Source: CAD feature listing. Evaluate the final solid. Frame: model axes, mm. A direction names the side the tool comes from. Give positions to 0.01 mm unless a question says otherwise; leave off trailing zeros. Write each loop counter-clockwise with the first axis right and the second up, starting at its lowest first coordinate (ties: lowest second). Pieces come first, ordered by that corner, then holes. Notation, with made-up numbers: (9.5, -24) -> (65.5, -24) arc R29 ccw to (65.5, 4) -> close; hole circle Ø7 at (-23, -13). An arc over 180 degrees is marked (long way). Write item = value, one per line.
from build123d import *

# Parameters (mm, degrees)
BOSS_EXTRUDE1_DEPTH = 10
SKETCH2_R           = 5
BOSS_EXTRUDE2_DEPTH = 30
CUT_EXTRUDE1_START  = 3.5
CUT_EXTRUDE1_DEPTH  = 4.5
CHAMFER1_SIZE       = 0.5


with BuildPart() as part:
    # Sketch1 → Boss-Extrude1 (new body)
    with BuildSketch(Plane.XY):
        with BuildLine():
            Line((-2, 7), (2, 7))
            Line((2, 7), (2, 4.582575695))
            ThreePointArc((2, 4.582575695), (0, -5), (-2, 4.582575695))
            Line((-2, 4.582575695), (-2, 7))
        make_face()
    extrude(amount=BOSS_EXTRUDE1_DEPTH)

    # Sketch2 → Boss-Extrude2 (add)
    with BuildSketch(Plane.XY.offset(10)):
        Circle(SKETCH2_R)
    extrude(amount=BOSS_EXTRUDE2_DEPTH)

    # Sketch3 → Cut-Extrude1 (cut, through all)
    with BuildSketch(Plane(origin=(0, 0, 0), x_dir=(1, 0, 0), z_dir=(0, 1, 0)).offset(CUT_EXTRUDE1_START)):
        with BuildLine():
            Line((1.5, -30), (1.5, -35))
            ThreePointArc((1.5, -35), (0, -36.5), (-1.5, -35))
            Line((-1.5, -35), (-1.5, -30))
            ThreePointArc((-1.5, -30), (0, -28.5), (1.5, -30))
        make_face()
    extrude(amount=CUT_EXTRUDE1_DEPTH, mode=Mode.SUBTRACT)

    # Chamfer1
    chamfer1_edges = [part.edges().sort_by_distance(p)[0] for p in [
        (-5, 0, 40),
    ]]
    chamfer(chamfer1_edges, length=CHAMFER1_SIZE)


solid = part.part
(1) Section query D-D (z = 32). Return loops of the section in (x, y).
Values follow:
outline = (-1.5, 3.5) -> (-1.5, 4.77) arc R5 ccw (long way) to (1.5, 4.77) -> (1.5, 3.5) -> close
(2) Pull-direction query (Z, two-part tool) for faces 1 (the face through (0, 0, 40)), 2 (the face through (0, 4.2, 36.5)), 3 (the face through (-2, 6, 5)); classes: pulls with the +Z half, pulls with the -Z half, needs draft (parallel to the pull), parting line crosses it, or undercut.
Values follow:
face_1 = pulls with the +Z half
face_2 = undercut
face_3 = needs draft
(3) Material intervals for line 1 (Z direction, x = 1.5, y = 5); line 2 (Y direction, x = 1, z = 12.5); line 3 (X direction, y = 1.5, z = 21), sorted ascending.
Values follow:
line_1 = 0 to 10
line_2 = -4.9 to 4.9
line_3 = -4.77 to 4.77
(4) Section query C-C (z = 27.5). Return loops of the section in (x, y), plus the area to 3 significant figures.
Values follow:
outline = circle Ø10 at (0, 0)
area = 78.5 mm2
(5) First-contact query: pin 1 (1 mm diameter, centred on y = 4, z = 32, fed in from +X); pin 2 (0.7 mm diameter, centred on y = 5.5, z = 6.5, fed in from +X); pin 3 (0.7 mm diameter, centred on x = 0.5, y = 5.5, fed in from +Z). Flat tips, straight axial feed; report the tip coordinate or a pass-through.
Values follow:
pin_1 = 3.57
pin_2 = 2
pin_3 = 10
(6) Section query A-A (x = 0). Return loops of the section in (y, z).
Values follow:
outline = (-5, 0) -> (7, 0) -> (7, 10) -> (5, 10) -> (5, 28.5) -> (3.5, 28.5) -> (3.5, 36.5) -> (5, 36.5) -> (5, 39.5) -> (4.5, 40) -> (-4.5, 40) -> (-5, 39.5) -> close
(7) Access query for faces 4 (the face through (0, 1, 0)), 5 (the face through (0, 3.5, 32)), 6 (the face through (2, 6, 5)). Directions: +Z, -Z, +X, -X, +Y, -Y. A direction counts if a zero-diameter tool reaches every point of the face in a straight line with its end or side. Return the directions, or none.
Values follow:
face_4 = -Z, +X, -X, +Y, -Y
face_5 = +Y
face_6 = +Z, -Z, +X, +Y
(8) Section query B-B (z = 8). Return loops of the section in (x, y), plus the area to 3 significant figures.
Values follow:
outline = (-2, 4.58) arc R5 ccw (long way) to (2, 4.58) -> (2, 7) -> (-2, 7) -> close
area = 87.1 mm2
